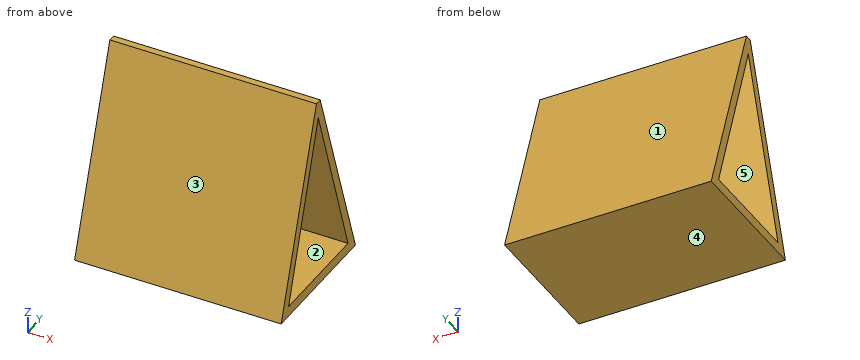
from build123d import *

# Parameters (mm, degrees)
PAD_DEPTH = 60


with BuildPart() as part:
    # Sketch → Pad (new body)
    with BuildSketch(Plane.YZ):
        Polygon((-20, 0), (20, 0), (1, 57), (-1, 57), align=None)
        Polygon((-16, 3), (16, 3), (0, 52), align=None, mode=Mode.SUBTRACT)
    extrude(amount=PAD_DEPTH)


solid = part.part
Read the model definition and answer for the solid it produces. Units are mm, in the model's axes. Face numbers are marked on the shaded views. A direction names the side the tool comes from. Coordinates: 2 decimals unless noted, no trailing zeros. Order: outer loops, then holes, each group sorted by start corner. A loop starts at its lowest first (then second) coordinate and runs counter-clockwise, first axis right, second up. Notation, with made-up numbers: M 82.25,21.5 L 139.25,21.5 A19 cw 139.25,26.5 Z; hole C -26.75,36 d11. An arc over 180 degrees is marked long. Put each result on its own line as item: value. Start each with the question number.
Item 1: Section D-D, the plane y = 18 is taken. Determine the outline of the cut face in (x, z), plus the area to 3 significant figures.
Item 2: Section C-C, the plane x = 25.5 is taken. Determine the outline of the cut face in (y, z), plus the area to 3 significant figures.
Item 3: Section A-A, the plane z = 17 is taken. Determine the outline of the cut face in (x, y), plus the area to 3 significant figures.
Item 4: Given pin 1 Ø6 at (x, z) = (17.5, 19) entering from +Y; pin 2 Ø2 at (x, z) = (15.5, 21.5) entering from +Y; pin 3 Ø12 at (x, z) = (20.5, 6.5) entering from -Y, each flat-ended and moving along its own axis, determine where each tip first touches the part or whether it passes through.
Item 5: The mould has two halves that part along Z. Classify the marked faces 3, 4 and 5: +Z half, -Z half, draft (parallel to the pull), parting line (faces both ways), or undercut.
Item 6: Section B-B, the plane y = -13 is taken. Determine the outline of the cut face in (x, z), plus the area to 3 significant figures.
Item 7: For the marked faces 1 and 2, determine the directions among +Z, -Z, +X, -X, +Y, -Y from which every point of the face is accessible in a straight line to the end or side of a thin tool.
Item 8: Consider probe 1 along Y at (x, z) = (31, 34.5); probe 2 along Y at (x, z) = (22.5, 23.5); probe 3 along Y at (x, z) = (12, 54). Determine where each line is inside the solid, lowest interval first. Write a range as [from, to].
Computed:
1. outline: M 0,0 L 60,0 L 60,6 L 0,6 Z
1. area: 360 mm2
2. outline: M -20,0 L 20,0 L 1,57 L -1,57 Z; hole M -16,3 L 16,3 L 0,52 Z
2. area: 413 mm2
3. outline: M 0,-14.33 L 60,-14.33 L 60,-11.43 L 0,-11.43 Z; M 0,11.43 L 60,11.43 L 60,14.33 L 0,14.33 Z
3. area: 349 mm2
4. pin 1: stops at y = 14.67
4. pin 2: stops at y = 13.17
4. pin 3: stops at y = -19.83
5. face 3: +Z half
5. face 4: -Z half
5. face 5: undercut
6. outline: M 0,0 L 60,0 L 60,3 L 0,3 Z; M 0,12.19 L 60,12.19 L 60,21 L 0,21 Z
6. area: 709 mm2
7. face 1: +Z, +X, -X, +Y
7. face 2: +X, -X
8. probe 1: y = [-8.5, -5.71], [5.71, 8.5]
8. probe 2: y = [-12.17, -9.31], [9.31, 12.17]
8. probe 3: y = [-2, 2]
